For this review, take the finished solid that the model builds, in its own axes (mm). Round coordinates to 2 decimals unless told otherwise and drop trailing zeros. Order: outer loops, then holes, each group sorted by start corner. A loop starts at its lowest first (then second) coordinate and runs counter-clockwise, first axis right, second up. Notation, with made-up numbers: M 46.25,82 L 73.25,82 A20 cw 73.25,97 Z; hole C -18,36 d1. An arc over 180 degrees is marked long. Answer in a Markdown table with one row per item. Add a question column.
Autodesk Inventor part; units mm, degrees
ref_plane "YZ Plane" through (0, 0, 0) normal (1, 0, 0) x (0, 1, 0)
ref_plane "XZ Plane" through (0, 0, 0) normal (0, 1, 0) x (-1, 0, 0)
ref_plane "XY Plane" through (0, 0, 0) normal (0, 0, 1) x (1, 0, 0)
sketch "Sketch1" plane through (0, 0, 0) normal (0, 0, 1) x (1, 0, 0)
  line L0 (0, 0) -> (12.7, 0)
  line L1 (12.7, 0) -> (12.7, 12.7)
  line L2 (12.7, 12.7) -> (0, 12.7)
  line L3 (0, 12.7) -> (0, 0)
  dimension "d0" = 12.7
  dimension "d1" = 12.7
extrude "Extrusion1" add sketch "Sketch1" along normal blind 80.01
sketch "Sketch2" plane through (12.7, 0, 0) normal (1, 0, 0) x (0, 0, -1)
  circle A0 centre (-43.815, 6.35) radius 5.715
  circle A1 centre (-36.195, 6.35) radius 5.715
  line L0 (-43.815, 6.35) -> (-36.195, 6.35) construction
  line L1 (0, 12.7) -> (-80.01, 12.7) construction
  line L2 (-36.195, 6.35) -> (-40.005, 6.35) construction
  line L3 (-80.01, 0) -> (-80.01, 12.7) construction
  point P0 (0, 0)
  point P1 (-40.005, 10.6097)
  point P2 (-40.005, 2.0903)
  dimension "d4" = 11.43
  dimension "d5" = 11.43
  dimension "d6" = 6.35
  dimension "d7" = 7.62
  dimension "d8" = 40.005
extrude "Extrusion2" cut sketch "Sketch2" against normal through all
sketch "Sketch3" plane through (0, 12.7, 0) normal (0, 1, 0) x (1, 0, 0)
  circle A0 centre (6.35, -75.311) radius 2
  line L0 (12.7, -80.01) -> (0, -80.01)
  line L1 (0, 0) -> (0, -80.01)
  circle A1 centre (6.35, -60.071) radius 2
  circle A2 centre (6.35, -4.699) radius 2
  circle A3 centre (6.35, -19.939) radius 2
  line L2 (12.7, 0) -> (0, 0)
  dimension "d11" = 4
  dimension "d12" = 4.699
  dimension "d13" = 6.35
  dimension "d14" = 4
  dimension "d15" = 15.24
  dimension "d16" = 6.35
  dimension "d17" = 4
  dimension "d18" = 4
  dimension "d19" = 6.35
  dimension "d20" = 6.35
  dimension "d21" = 4.699
  dimension "d22" = 15.24
extrude "Extrusion3" cut sketch "Sketch3" against normal through all
properties part number "Mockup Load Cell (based on 1kg Adafruit)"
1. Clearance check with a flat-ended pin moving along its axis: pin 1 Ø2.5 at (x, z) = (6.35, 75.311) entering from +Y. State where the tip first meets the part, or that it passes through.
2. Consider section A-A on y = 6.35. Write out the cut boundary in (x, z).
3. Consider section C-C on y = 3.25. Write out the cut boundary in (x, z), plus the area to 3 significant figures.
4. Consider section B-B on x = 6.35. Write out the cut boundary in (y, z) (3 decimals), plus the area to 3 significant figures.
5. To check wall thickness, follow probe 1 along Z at (x, y) = (6.35, 9.25); probe 2 along Z at (x, y) = (5.25, 12.25); probe 3 along Z at (x, y) = (7, 5.5). State the ranges of each line that lie inside material, in increasing order. Write a range as [from, to].
6. The part is to be moulded in two halves that separate along X. For faces 1 (the cylindrical face through (5.916, 6.439, 77.263)), 2 (the flat face through (12.7, 12, 39)), 3 (the flat face through (6, 12.7, 39)), 4 (the cylindrical face through (6.09, 6.439, 58.088)), say which applies: pulls with the +X half, pulls with the -X half, needs draft (parallel to the pull), parting line crosses it, or undercut.
Solved:
| question | item | result |
|---|---|---|
| 1 | pin 1 | passes through |
| 2 | outline | M 0,0 L 12.7,0 L 12.7,30.48 L 0,30.48 Z; M 0,49.53 L 12.7,49.53 L 12.7,80.01 L 0,80.01 Z; hole C 6.35,4.7 d4; hole C 6.35,19.94 d4; hole C 6.35,60.07 d4; hole C 6.35,75.31 d4 |
| 3 | outline | M 0,0 L 12.7,0 L 12.7,31.39 L 0,31.39 Z; M 0,48.62 L 12.7,48.62 L 12.7,80.01 L 0,80.01 Z; hole C 6.35,4.7 d4; hole C 6.35,19.94 d4; hole C 6.35,60.07 d4; hole C 6.35,75.31 d4 |
| 3 | area | 747 mm^2 |
| 4 | outline | M 0,0 L 12.7,0 L 12.7,2.699 L 0,2.699 Z; M 0,6.699 L 12.7,6.699 L 12.7,17.939 L 0,17.939 Z; M 0,21.939 L 12.7,21.939 L 12.7,58.071 L 0,58.071 Z; M 0,62.071 L 12.7,62.071 L 12.7,73.311 L 0,73.311 Z; M 0,77.311 L 12.7,77.311 L 12.7,80.01 L 0,80.01 Z; hole M 2.09,40.005 A5.715 ccw long 10.61,40.005 A5.715 ccw long Z |
| 4 | area | 630 mm^2 |
| 5 | probe 1 | z = [0, 2.7], [6.7, 17.94], [21.94, 31.27], [48.74, 58.07], [62.07, 73.31], [77.31, 80.01] |
| 5 | probe 2 | z = [0, 3.03], [6.37, 18.27], [21.61, 58.4], [61.74, 73.64], [76.98, 80.01] |
| 5 | probe 3 | z = [0, 2.81], [6.59, 18.05], [21.83, 30.54], [49.47, 58.18], [61.96, 73.42], [77.2, 80.01] |
| 6 | face 1 | undercut |
| 6 | face 2 | pulls with the +X half |
| 6 | face 3 | needs draft |
| 6 | face 4 | undercut |
